CAD build for the part. Positions are in the model's coordinates, mm. Face numbers are marked on the shaded views. A direction names the side the tool comes from. Give positions to 0.01 mm unless a question says otherwise; leave off trailing zeros. Write each loop counter-clockwise with the first axis right and the second up, starting at its lowest first coordinate (ties: lowest second). Pieces come first, ordered by that corner, then holes. Notation, with made-up numbers: (22, 88) - (46, 88) arc R27 ccw to (46, 114) - close; hole circle Ø11 at (78, 86.25). An arc over 180 degrees is marked (long way). Answer as a JSON object with one key per item and string values.
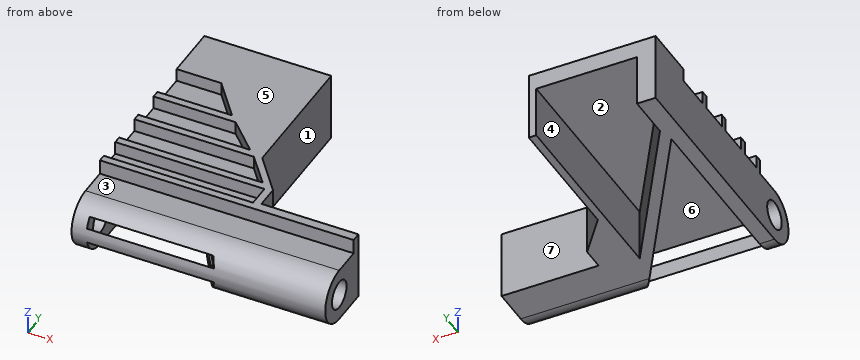
from build123d import *

# Parameters (mm, degrees)
PAD_DEPTH       = 68
SKETCH001_R     = 3.8
POCKET_DEPTH    = 68.001
POCKET001_DEPTH = 18.601
SKETCH003_W     = 6
SKETCH003_H     = 40
POCKET002_DEPTH = 3.5
POCKET003_DEPTH = 12
POCKET004_DEPTH = 14


with BuildPart() as part:
    # Sketch → Pad (new body)
    with BuildSketch(Plane.YZ):
        with BuildLine():
            ThreePointArc((0, 14.6), (-7.3, 7.3), (0, 0))
            Line((0, 0), (62, 0))
            Line((62, 0), (62, 18.6))
            Line((7.5, 18.6), (62, 18.6))
            Line((7.5, 14.6), (7.5, 18.6))
            Line((0, 14.6), (7.5, 14.6))
        make_face()
    extrude(amount=PAD_DEPTH)

    # Sketch001 (on Face8 of Pad) → Pocket (cut, through all)
    with BuildSketch(Plane.YZ.offset(68)):
        with Locations((0, 7.3)):
            Circle(SKETCH001_R)
    extrude(amount=-POCKET_DEPTH, mode=Mode.SUBTRACT)

    # Sketch002 (on Face8 of Pocket) → Pocket001 (cut, through all)
    with BuildSketch(Plane(origin=(0, 0, 18.6), x_dir=(0, -1, 0), z_dir=(0, 0, 1))):
        Polygon((-62, 34), (-26, 34), (-16, 42), (-10, 42), (-10, 68), (-62, 68), align=None)
    extrude(amount=-POCKET001_DEPTH, mode=Mode.SUBTRACT)

    # Sketch003 (on Face12 of Pocket001) → Pocket002 (cut)
    with BuildSketch(Plane(origin=(0, 0, 18.6), x_dir=(0, -1, 0), z_dir=(0, 0, 1))):
        with Locations((-12.5, 20)):
            Rectangle(SKETCH003_W, SKETCH003_H)
        Polygon((-25.5, 0), (-25.5, 32), (-17.5, 38.5), (-17.5, 0), align=None)
        Polygon((-35.5, 0), (-35.5, 22), (-27.5, 30), (-27.5, 0), align=None)
        Polygon((-47.5, 0), (-47.5, 12), (-37.5, 20), (-37.5, 0), align=None)
    extrude(amount=-POCKET002_DEPTH, mode=Mode.SUBTRACT)

    # Sketch004 (on Face3 of Pocket002) → Pocket003 (cut)
    with BuildSketch(Plane.YX):
        Polygon((-7, 38), (-7, 4), (46, 4), align=None)
    extrude(amount=-POCKET003_DEPTH, mode=Mode.SUBTRACT)

    # Sketch005 (on Face3 of Pocket003) → Pocket004 (cut)
    with BuildSketch(Plane.YX):
        Polygon((8, 32), (62, 32), (62, 5), (50, 5), align=None)
    extrude(amount=-POCKET004_DEPTH, mode=Mode.SUBTRACT)


solid = part.part
Item 1: Cut at D-D (z = 7.3). Give the cut face in (x, y), and give its area (3 significant figures).
Entries:
{"outline": "(0, -7.3) - (68, -7.3) - (68, -3.8) - (35.95, -3.8) - (38, -7) - (4, -7) - (4, -3.8) - (0, -3.8) - close; (0, 3.8) - (4, 3.8) - (4, 46) - (31.07, 3.8) - (68, 3.8) - (68, 10) - (42, 10) - (42, 16) - (34, 26) - (34, 62) - (32, 62) - (32, 8) - (5, 50) - (5, 62) - (0, 62) - close", "area": "948 mm2"}
Item 2: Flat gauge pins, fed straight in: P1, Ø3.5, axis at x = 18, z = 8, coming from the +Y side; P2, Ø6, axis at x = 11, z = 8, coming from the +Y side; P3, Ø1.8, axis at y = 12.5, z = 16.5, coming from the -X side; P4, Ø7, axis at y = 0, z = 7.3, coming from the +X side. Where does each tip first touch, or does it go through?
Entries:
{"P1": "y = 32.5", "P2": "y = 45.33", "P3": "x = 40", "P4": "through"}
Item 3: Mould opens along X. For the marked faces 1, 2 and 3 say: +X half, -X half, draft (parallel to the pull), parting line (faces both ways), or undercut.
Entries:
{"face 1": "+X half", "face 2": "undercut", "face 3": "draft"}
Item 4: Cut at B-B (y = 51). Give the cut face in (x, z).
Entries:
{"outline": "(0, 0) - (5, 0) - (5, 14) - (32, 14) - (32, 0) - (34, 0) - (34, 18.6) - (0, 18.6) - close"}
Item 5: Cut at C-C (x = 25). Give the cut face in (y, z), and give its area (3 significant figures).
Entries:
{"outline": "(-7, 5.23) - (-7, 9.37) arc R7.3 ccw to start; (-5.59, 12) - (13.26, 12) - (13.26, 0) - (18.89, 0) - (18.89, 14) - (62, 14) - (62, 18.6) - (32.5, 18.6) - (32.5, 15.1) - (27.5, 15.1) - (27.5, 18.6) - (25.5, 18.6) - (25.5, 15.1) - (17.5, 15.1) - (17.5, 18.6) - (15.5, 18.6) - (15.5, 15.1) - (9.5, 15.1) - (9.5, 18.6) - (7.5, 18.6) - (7.5, 14.6) - (0, 14.6) arc R7.3 ccw to start", "area": "305 mm2"}
Item 6: Cut at A-A (z = 16.5). Give the cut face in (x, y).
Entries:
{"outline": "(0, 7.5) - (68, 7.5) - (68, 10) - (42, 10) - (42, 16) - (34, 26) - (34, 62) - (0, 62) - (0, 47.5) - (12, 47.5) - (20, 37.5) - (0, 37.5) - (0, 35.5) - (22, 35.5) - (30, 27.5) - (0, 27.5) - (0, 25.5) - (32, 25.5) - (38.5, 17.5) - (0, 17.5) - (0, 15.5) - (40, 15.5) - (40, 9.5) - (0, 9.5) - close"}
Item 7: Which spindle directions (+Z, -Z, +X, -X, +Y, -Y) get a long thin tool onto all of the face, cutting with end or side? Do the marked faces 4, 5, 6 and 7. Say none if no direction does.
Entries:
{"face 4": "-Z, +Y", "face 5": "+Z, +X, -X, +Y, -Y", "face 6": "-Z, -Y", "face 7": "+Z, -Z, +X, +Y"}
Item 8: Probe line 1 (Y direction, x = 6, z = 17); line 2 (Y direction, x = 51.5, z = 7.3); line 3 (Z direction, x = 1.85, y = 0). List the from-to ranges inside material, lowest first. Write a range as from..to.
Entries:
{"line 1": "7.5..9.5, 15.5..17.5, 25.5..27.5, 35.5..37.5, 47.5..62", "line 2": "-7.3..-3.8, 3.8..10", "line 3": "0..3.5, 11.1..14.6"}
